Part model, mm, in its own coordinate system. Face numbers are marked on the shaded views. A direction names the side the tool comes from. Coordinates: 2 decimals unless noted, no trailing zeros. Loops run counter-clockwise (first coordinate to the right, second up) from the corner with the lowest first, then second, coordinate; pieces in that order, holes last. Notation, with made-up numbers: (-26.75, 3) -> (-2.75, 3) arc R17 cw to (-2.75, 11) -> close; hole circle Ø2 at (16.25, 60). An arc over 180 degrees is marked (long way). Use one line per item in the form item = value. Start each with the question number.
(1) Band-saw the part on C-C on z = -1.75. Give the cut face in (x, y) (3 decimals), then the cut area to 3 significant figures.
(2) Band-saw the part on B-B on y = 5.5. Give the cut face in (x, z) (3 decimals), then the cut area to 3 significant figures.
(3) Mould opens along Y. For the marked faces 1, 2 and 3 say: +Y half, -Y half, draft (parallel to the pull), parting line (faces both ways), or undercut.
(4) Pin check, flat tip, straight feed: P1, Ø3, axis at x = -12, z = 2.5, coming from the +Y side. Stop position of the tip, or through.
(5) Drill centre lines: L1, parallel to X at y = -2.5, z = 2.25; L2, parallel to X at y = 0.5, z = 0.5; L3, parallel to X at y = 10, z = 0.5. Where is each one in solid material? Low to high. Write a range as [from, to].
(6) 3-axis set-ups, long thin cutter, end or side, ignore diameter. For the marked faces 4 and 5: which of +Z, -Z, +X, -X, +Y, -Y reach the whole face in a straight line?
(7) Band-saw the part on A-A on y = 0. Give the cut face in (x, z) (3 decimals).
(8) Band-saw the part on D-D on x = 0. Give the cut face in (y, z) (3 decimals), then the cut area to 3 significant figures.
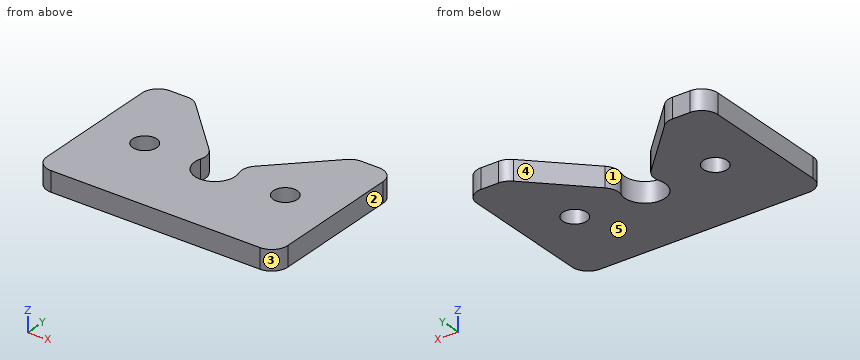
```python
from build123d import *

# Parameters (mm, degrees)
F1_DEPTH = 3.175
F2_R     = 5.08
F3_R     = 3.81
F4_DEPTH = 25.4


with BuildPart() as f1:
    # F0 (on Top) → F1 (new body, symmetric)
    with BuildSketch(Plane.XY):
        with BuildLine():
            Line((-38.1, -25.4), (38.1, -25.4))
            Line((38.1, -25.4), (38.1, 25.4))
            Line((38.1, 25.4), (25.4, 25.4))
            Line((25.4, 25.4), (4.4901280605, 4.4901280605))
            ThreePointArc((4.4901280605, 4.4901280605), (0, -6.35), (-4.4901280605, 4.4901280605))
            Line((-4.4901280605, 4.4901280605), (-25.4, 25.4))
            Line((-25.4, 25.4), (-38.1, 25.4))
            Line((-38.1, 25.4), (-38.1, -25.4))
        make_face()
    extrude(amount=F1_DEPTH, both=True)

    # F2
    f2_edges = [f1.edges().sort_by_distance(p)[0] for p in [
        (4.490128, 4.490128, 0),
        (-4.490128, 4.490128, 0),
        (-25.4, 25.4, 0),
        (-38.1, 25.4, 0),
        (-38.1, -25.4, 0),
        (38.1, 25.4, 0),
        (25.4, 25.4, 0),
        (38.1, -25.4, 0),
    ]]
    fillet(f2_edges, radius=F2_R)

    # F3 (on face) → F4 (cut)
    with BuildSketch(Plane.XY.offset(3.175)):
        with BuildLine():
            ThreePointArc((-26.035, 0), (-22.225, -3.81), (-18.415, 0))
            ThreePointArc((-18.415, 0), (-22.225, 3.81), (-26.035, 0))
        make_face()
        with Locations((22.225, 0)):
            Circle(F3_R)
    extrude(amount=-F4_DEPTH, mode=Mode.SUBTRACT)


solid = f1.part
```
A:
q1.outline = (-38.1, -20.32) arc R5.08 ccw to (-33.02, -25.4) -> (33.02, -25.4) arc R5.08 ccw to (38.1, -20.32) -> (38.1, 20.32) arc R5.08 ccw to (33.02, 25.4) -> (27.504, 25.4) arc R5.08 ccw to (23.912, 23.912) -> (7.24, 7.24) arc R5.08 ccw to (6.018, 2.027) arc R6.35 cw (long way) to (-6.018, 2.027) arc R5.08 ccw to (-7.24, 7.24) -> (-23.912, 23.912) arc R5.08 ccw to (-27.504, 25.4) -> (-33.02, 25.4) arc R5.08 ccw to (-38.1, 20.32) -> close; hole circle Ø7.62 at (-22.225, 0); hole circle Ø7.62 at (22.225, 0)
q1.area = 3,010 mm²
q2.outline = (-38.1, -3.175) -> (-6.102, -3.175) -> (-6.102, 3.175) -> (-38.1, 3.175) -> close; (6.102, -3.175) -> (38.1, -3.175) -> (38.1, 3.175) -> (6.102, 3.175) -> close
q2.area = 406 mm²
q3.face_1 = undercut
q3.face_2 = draft
q3.face_3 = -Y half
q4.P1 = 13.5
q5.L1 = [-38.1, -25.1], [-19.35, -5.84], [5.84, 19.35], [25.1, 38.1]
q5.L2 = [-38.1, -26], [-18.45, -6.33], [6.33, 18.45], [26, 38.1]
q5.L3 = [-38.1, -10], [10, 38.1]
q6.face_4 = +Z, -Z, +Y
q6.face_5 = -Z, +X, -X, +Y, -Y
q7.outline = (-38.1, -3.175) -> (-26.035, -3.175) -> (-26.035, 3.175) -> (-38.1, 3.175) -> close; (-18.415, -3.175) -> (-6.35, -3.175) -> (-6.35, 3.175) -> (-18.415, 3.175) -> close; (6.35, -3.175) -> (18.415, -3.175) -> (18.415, 3.175) -> (6.35, 3.175) -> close; (26.035, -3.175) -> (38.1, -3.175) -> (38.1, 3.175) -> (26.035, 3.175) -> close
q8.outline = (-25.4, -3.175) -> (-6.35, -3.175) -> (-6.35, 3.175) -> (-25.4, 3.175) -> close
q8.area = 121 mm²
